Geometry: see drawing. Coordinates: mm, zero at the bounding-box minimum. A direction names the side the tool comes from. Coordinates: 2 decimals unless noted, no trailing zeros. Loops run counter-clockwise (first coordinate to the right, second up) from the corner with the lowest first, then second, coordinate; pieces in that order, holes last. Notation, with made-up numbers: (-31.5, 27) -> (9.5, 27) arc R19 cw to (9.5, 40) -> close; hole circle Ø7 at (-23.75, 71.5). An arc over 180 degrees is marked (long way). One line per item, written item: value. Start each with the question number.
Item 1: Contact query for flat-ended pins moving along their axis: pin 1 Ø6 at (x, z) = (5, 26.5) entering from -Y; pin 2 Ø8 at (y, z) = (20, 13.5) entering from +X; pin 3 Ø1.5 at (x, z) = (11.5, 22) entering from +Y; pin 4 Ø10 at (x, y) = (8, 4.5) entering from -Z. Output: stop coordinate, or through.
Item 2: Ray query, probe 1 along Z at (x, y) = (26, 8); probe 2 along Y at (x, z) = (19, 10); probe 3 along Y at (x, z) = (26.5, 24.5). Return the intervals inside material, ascending. Write a range as from..to.
Item 3: Set-up query: the marked faces 1 and 2. Return all of +Z, -Z, +X, -X, +Y, -Y with unobstructed straight access to the full face (end or side cutting, diameter ignored); none if empty.
Item 4: Section query D-D on y = 28.5. Return loops of the section in (x, z).
Item 5: Section query C-C on z = 24.5. Return loops of the section in (x, y), then the cut area to 3 significant figures.
Item 6: Section query A-A on y = 15.24. Return loops of the section in (x, z).
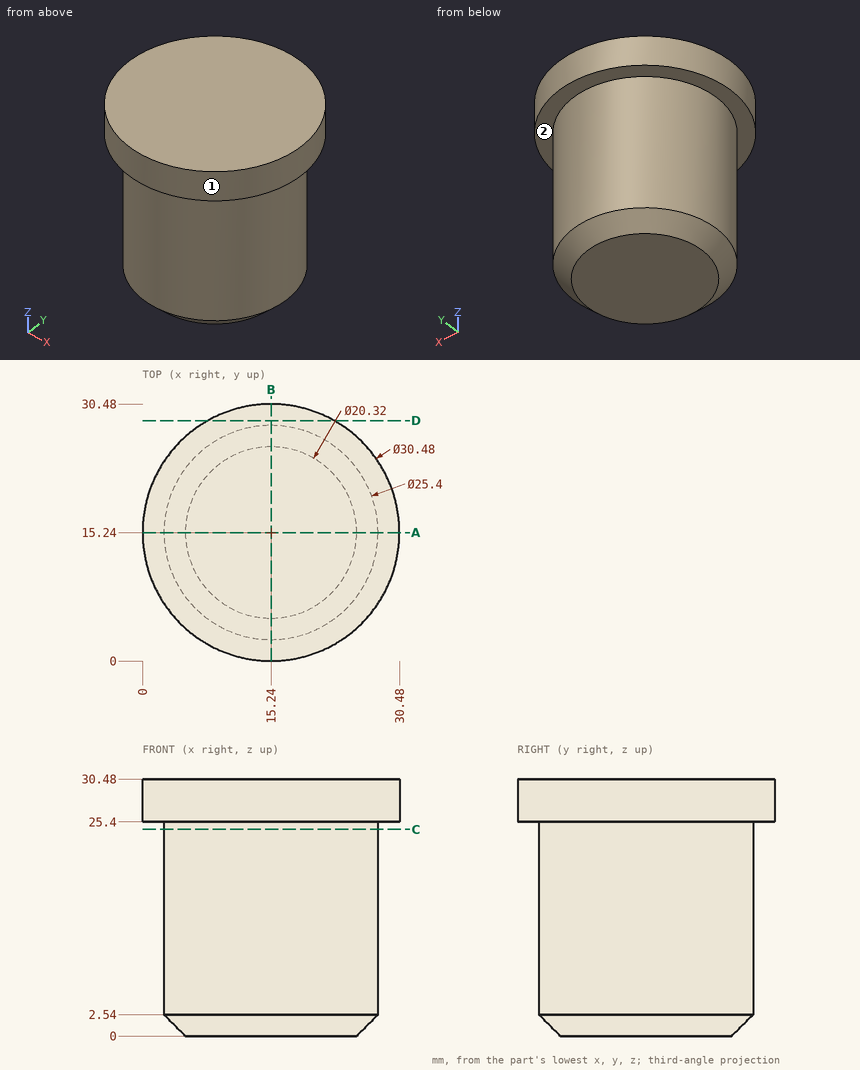
Reply:
1. pin 1: stops at y = 1.83
1. pin 2: stops at x = 27.92
1. pin 3: stops at y = 27.58
1. pin 4: stops at z = 0
2. probe 1: z = 25.4..30.48
2. probe 2: y = 3.11..27.37
2. probe 3: y = 9.37..21.11
3. face 1: +Z, -Z
3. face 2: -Z
4. outline: (7.73, 25.4) -> (22.75, 25.4) -> (22.75, 30.48) -> (7.73, 30.48) -> close
5. outline: circle Ø25.4 at (15.24, 15.24)
5. area: 507 mm²
6. outline: (0, 25.4) -> (2.54, 25.4) -> (2.54, 2.54) -> (5.08, 0) -> (25.4, 0) -> (27.94, 2.54) -> (27.94, 25.4) -> (30.48, 25.4) -> (30.48, 30.48) -> (0, 30.48) -> close
